The model under review builds one solid part; all positions refer to its coordinate system, in mm. A direction names the side the tool comes from. Give positions to 0.01 mm unless a question says otherwise; leave off trailing zeros. Write each loop counter-clockwise with the first axis right and the second up, starting at its lowest first coordinate (ties: lowest second). Pieces come first, ordered by that corner, then holes. Notation, with made-up numbers: M 74.5,7.5 L 116.5,7.5 A11 ccw 116.5,26.5 Z; hole C 3.5,-34.5 d4. An arc over 180 degrees is marked long. Write item = value, one per line. Start each with the question number.
```python
from build123d import *

# Parameters (mm, degrees)
BOSS_EXTRUDE1_DEPTH = 34.925
SKETCH2_R           = 2.921
CUT_EXTRUDE1_DEPTH  = 99.014466407
SKETCH4_W           = 50.8
SKETCH4_H           = 28.575
CUT_EXTRUDE3_DEPTH  = 99.014466407
FILLET1_R           = 5.08
SKETCH5_R           = 4.318
CUT_EXTRUDE4_DEPTH  = 12.7


with BuildPart() as part:
    # Sketch1 → Boss-Extrude1 (new body)
    with BuildSketch(Plane.XY):
        Polygon((0, 0), (0, 50.8), (25.4, 50.8), (25.4, 25.4), (76.2, 25.4), (76.2, 0), align=None)
    extrude(amount=BOSS_EXTRUDE1_DEPTH)

    # Sketch2 → Cut-Extrude1 (cut, through all)
    with BuildSketch(Plane.XY.offset(34.925)):
        with Locations((12.7, 38.1)):
            Circle(SKETCH2_R)
        with Locations((12.7, 12.7)):
            Circle(SKETCH2_R)
        with Locations((38.1, 12.7)):
            Circle(SKETCH2_R)
        with Locations((63.5, 12.7)):
            Circle(SKETCH2_R)
    extrude(amount=-CUT_EXTRUDE1_DEPTH, mode=Mode.SUBTRACT)

    # Sketch4 → Cut-Extrude3 (cut, through all)
    with BuildSketch(Plane.XZ):
        with Locations((50.8, 14.2875)):
            Rectangle(SKETCH4_W, SKETCH4_H)
    extrude(amount=-CUT_EXTRUDE3_DEPTH, mode=Mode.SUBTRACT)

    # Fillet1
    fillet1_edges = [part.edges().sort_by_distance(p)[0] for p in [
        (25.4, 25.4, 31.75),
        (25.4, 12.7, 28.575),
    ]]
    fillet(fillet1_edges, radius=FILLET1_R)

    # Sketch5 → Cut-Extrude4 (cut)
    with BuildSketch(Plane.XY.offset(34.925)):
        with Locations((12.7, 38.1)):
            Circle(SKETCH5_R)
    extrude(amount=-CUT_EXTRUDE4_DEPTH, mode=Mode.SUBTRACT)


solid = part.part
```
Item 1: For faces 4 (the flat face through (25.4, 25, 13)), 5 (the flat face through (53, 13, 28.575)), 6 (the flat face through (16, 37, 22.225)), list the 3-axis set-ups (+Z, -Z, +X, -X, +Y, -Y) from which the entire face can be reached by the end or side of a thin tool; tool diameter is ignored.
Item 2: We need section A-A, the plane x = 63.5. Write out the cut boundary in (y, z) (3 decimals), and give its area (3 significant figures).
Item 3: To check wall thickness, follow probe 1 along Y at (x, z) = (12.7, 31.75); probe 2 along Y at (x, z) = (13, 13); probe 3 along Y at (x, z) = (38, 33). State the ranges of each line that lie inside material, in increasing order. Write a range as [from, to].
Item 4: We need section D-D, the plane y = 11.5. Write out the cut boundary in (x, z) (3 decimals), and give its area (3 significant figures).
Item 5: The part is to be moulded in two halves that separate along Y. For faces 1 (the cylindrical face through (12.14, 42.38, 28.66)), 2 (the flat face through (13, 50.8, 17)), 3 (the flat face through (13, 26, 0)), say which applies: released by +Y, released by -Y, zero draft, split by the parting line, or undercut.
Item 6: We need section C-C, the plane z = 17.5. Write out the cut boundary in (x, y).
Item 7: Clearance check with flat-ended pins moving along their axes: P1, Ø12, axis at x = 38.5, z = 23, coming from the +Y side; P2, Ø9.5, axis at x = 38.1, y = 12.7, coming from the -Z side (3 decimals); P3, Ø2.5, axis at x = 11, y = 40, coming from the +Z side (3 decimals). State where each tip first meets the part, or that it passes through.
Item 8: We need section B-B, the plane y = 38.1. Write out the cut boundary in (x, z) (3 decimals), and give its area (3 significant figures).
Worked out:
q1.face_4 = -Z, +X, +Y
q1.face_5 = -Z, +X, +Y, -Y
q1.face_6 = +Z
q2.outline = M 0,28.575 L 9.779,28.575 L 9.779,34.925 L 0,34.925 Z; M 15.621,28.575 L 25.4,28.575 L 25.4,34.925 L 15.621,34.925 Z
q2.area = 124 mm²
q3.probe_1 = [0, 9.78], [15.62, 33.78], [42.42, 50.8]
q3.probe_2 = [0, 9.79], [15.61, 35.19], [41.01, 50.8]
q3.probe_3 = [0, 9.78], [15.62, 25.4]
q4.outline = M 0,0 L 10.037,0 L 10.037,34.925 L 0,34.925 Z; M 15.363,0 L 25.4,0 L 25.4,23.495 A5.08 cw 30.48,28.575 L 35.437,28.575 L 35.437,34.925 L 15.363,34.925 Z; M 40.763,28.575 L 60.837,28.575 L 60.837,34.925 L 40.763,34.925 Z; M 66.163,28.575 L 76.2,28.575 L 76.2,34.925 L 66.163,34.925 Z
q4.area = 962 mm²
q5.face_1 = undercut
q5.face_2 = released by +Y
q5.face_3 = zero draft
q6.outline = M 0,0 L 25.4,0 L 25.4,50.8 L 0,50.8 Z; hole C 12.7,12.7 d5.84; hole C 12.7,38.1 d5.84
q7.P1 = 25.4
q7.P2 = 28.575
q7.P3 = 22.225
q8.outline = M 0,0 L 9.779,0 L 9.779,22.225 L 8.382,22.225 L 8.382,34.925 L 0,34.925 Z; M 15.621,0 L 25.4,0 L 25.4,34.925 L 17.018,34.925 L 17.018,22.225 L 15.621,22.225 Z
q8.area = 648 mm²
